Can you work these out from the model? Positions are in its coordinate system, mm. Face numbers are marked on the shaded views. Round coordinates to 2 decimals unless told otherwise and drop trailing zeros. Loops run counter-clockwise (first coordinate to the right, second up) from the corner with the lowest first, then second, coordinate; pieces in that order, holes last.
(1) I want a section at A-A on y = 1.5. Write out the boundary of the cut face in (x, z), plus the area to 3 significant figures.
(2) I want a section at B-B on z = 0. Give the number of separate pieces and of enclosed holes in the cut face, plus the area to 3 significant figures.
(3) If I drill on line 1 along X through (y, z) = (1.35, 0); line 2 along X through (y, z) = (0.7, 0.75); line 3 along Z through (x, y) = (14, 0.25), over which ranges is the centre line in solid material (lowest first)?
(4) Thinking about a two-plate mould opening in Z: for the marked faces 1, 2 and 3, which applies, released by +Z, released by -Z, zero draft, split by the parting line, or undercut?
(5) Will these pins go through, and if not, where does the flat tip stop? pin 1 Ø1.5 at (y, z) = (1, -2.5) entering from +X; pin 2 Ø3 at (x, z) = (14.38, -0.8) entering from +Y; pin 3 Ø1 at (x, y) = (6, 2.5) entering from +Z.
from build123d import *

# Parameters (mm, degrees)
SKETCH_1_R      = 1.75
EXTRUDE_1_DEPTH = 3
CHAMFER_1_SIZE  = 0.3


with BuildPart() as part:
    # 草图1 → 凸台-拉伸1 (new body)
    with BuildSketch(Plane(origin=(0, 0, 0), x_dir=(1, 0, 0), z_dir=(0, 1, 0))):
        with BuildLine():
            Line((-8.058099854, 3.286572102), (-8.934273675, 1.52529864))
            ThreePointArc((-8.934273675, 1.52529864), (-9.030809196, -0.481724252), (-7.6190352, -1.911533393))
            ThreePointArc((-7.6190352, -1.911533393), (4.381181498, -4.208142868), (16.381398197, -1.911533393))
            ThreePointArc((16.381398197, -1.911533393), (17.793172193, -0.481724252), (17.696636672, 1.52529864))
            Line((17.696636672, 1.52529864), (16.820462851, 3.286572102))
            ThreePointArc((16.820462851, 3.286572102), (15.733455475, 4.267905138), (14.26918179, 4.245496696))
            ThreePointArc((14.26918179, 4.245496696), (4.381181498, 2.291857132), (-5.506818793, 4.245496696))
            ThreePointArc((-5.506818793, 4.245496696), (-6.971092478, 4.267905138), (-8.058099854, 3.286572102))
        make_face()
        with Locations(Location((-5.618818502, 0.804359974, 0), (0, 0, 270))):
            Circle(SKETCH_1_R, mode=Mode.SUBTRACT)
        with Locations(Location((14.381181498, 0.804359974, 0), (0, 0, 270))):
            Circle(SKETCH_1_R, mode=Mode.SUBTRACT)
    extrude(amount=EXTRUDE_1_DEPTH)

    # 倒角1
    chamfer_1_edges = [part.edges().sort_by_distance(p)[0] for p in [
        (4.381181498, 0, -2.291857132),
        (15.733455475, 0, -4.267905138),
        (17.258549762, 0, -2.405935371),
        (17.793172193, 0, 0.481724252),
        (15.733455475, 3, -4.267905138),
        (4.381181498, 3, -2.291857132),
        (-6.971092478, 3, -4.267905138),
        (-5.618818502, 0, -2.554359974),
        (-5.618818502, 3, -2.554359974),
        (-8.496186765, 3, -2.405935371),
        (14.381181498, 0, -2.554359974),
        (14.381181498, 3, -2.554359974),
        (-9.030809196, 3, 0.481724252),
        (4.381181498, 3, 4.208142868),
        (17.793172193, 3, 0.481724252),
        (4.381181498, 0, 4.208142868),
        (17.258549762, 3, -2.405935371),
        (-9.030809196, 0, 0.481724252),
        (-8.496186765, 0, -2.405935371),
        (-6.971092478, 0, -4.267905138),
    ]]
    chamfer(chamfer_1_edges, length=CHAMFER_1_SIZE)


solid = part.part
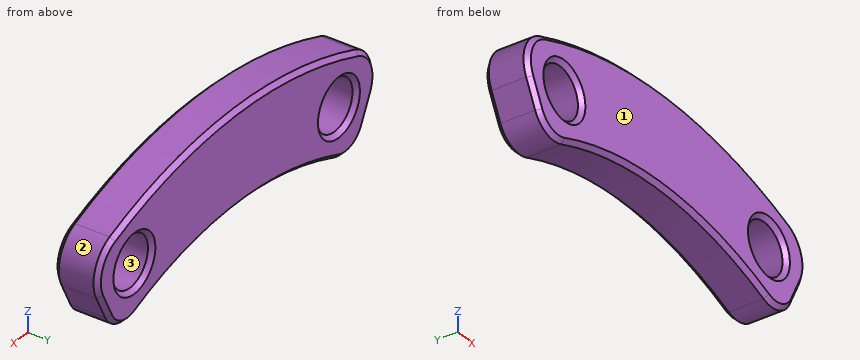
Filled sheet:
1. outline: (-8.93, -1.53) - (-8.06, -3.29) arc R2 ccw to (-5.51, -4.25) arc R26 cw to (14.27, -4.25) arc R2 ccw to (16.82, -3.29) - (17.7, -1.53) arc R2.5 ccw to (16.38, 1.91) arc R32.5 ccw to (-7.62, 1.91) arc R2.5 ccw to start; hole circle Ø3.5 at (-5.62, -0.8); hole circle Ø3.5 at (14.38, -0.8)
1. area: 152 mm2
2. separate pieces: 3
2. enclosed holes: 0
2. area: 62.0 mm2
3. line 1: x = -9.16 to -7.17, -4.06 to 12.83, 15.94 to 17.92
3. line 2: x = -8.91 to -6.42, -4.81 to 13.58, 15.19 to 17.67
3. line 3: z = -4.08 to -2.56, 0.95 to 2.7
4. face 1: zero draft
4. face 2: split by the parting line
4. face 3: undercut
5. pin 1: stops at x = 17.58
5. pin 2: passes through
5. pin 3: stops at z = 4.19
